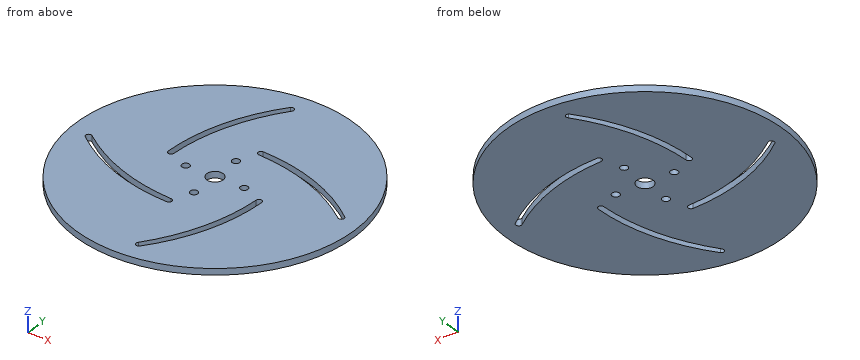
```python
from build123d import *

# Parameters (mm, degrees)
SKETCH1_R           = 69.85
SKETCH1_R_2         = 4.1
BOSS_EXTRUDE1_DEPTH = 3.175
SKETCH4_R           = 1.905
CUT_EXTRUDE1_DEPTH  = 4.175


with BuildPart() as part:
    # Sketch1 → Boss-Extrude1 (new body)
    with BuildSketch(Plane.XY):
        Circle(SKETCH1_R)
        Circle(SKETCH1_R_2, mode=Mode.SUBTRACT)
        with BuildLine():
            ThreePointArc((60.715904818, 5.788404818), (34.486591453, 20.94201271), (4.777601385, 26.856792578))
            ThreePointArc((4.777601385, 26.856792578), (3.305570957, 25.407474231), (4.762499202, 23.942975224))
            ThreePointArc((4.762499202, 23.942975224), (33.266012569, 17.981736248), (58.664095182, 3.736595182))
            ThreePointArc((58.664095182, 3.736595182), (60.715904818, 3.736595182), (60.715904818, 5.788404818))
        make_face(mode=Mode.SUBTRACT)
        with BuildLine():
            ThreePointArc((-23.942975224, 4.762499202), (-17.981736248, 33.266012569), (-3.736595182, 58.664095182))
            ThreePointArc((-3.736595182, 58.664095182), (-3.736595182, 60.715904818), (-5.788404818, 60.715904818))
            ThreePointArc((-5.788404818, 60.715904818), (-20.94201271, 34.486591453), (-26.856792578, 4.777601385))
            ThreePointArc((-26.856792578, 4.777601385), (-25.407474231, 3.305570957), (-23.942975224, 4.762499202))
        make_face(mode=Mode.SUBTRACT)
        with BuildLine():
            ThreePointArc((5.788404818, -60.715904818), (20.94201271, -34.486591453), (26.856792578, -4.777601385))
            ThreePointArc((26.856792578, -4.777601385), (25.407474231, -3.305570957), (23.942975224, -4.762499202))
            ThreePointArc((23.942975224, -4.762499202), (17.981736248, -33.266012569), (3.736595182, -58.664095182))
            ThreePointArc((3.736595182, -58.664095182), (3.736595182, -60.715904818), (5.788404818, -60.715904818))
        make_face(mode=Mode.SUBTRACT)
        with BuildLine():
            ThreePointArc((-60.715904818, -5.788404818), (-34.486591453, -20.94201271), (-4.777601385, -26.856792578))
            ThreePointArc((-4.777601385, -26.856792578), (-3.305570957, -25.407474231), (-4.762499202, -23.942975224))
            ThreePointArc((-4.762499202, -23.942975224), (-33.266012569, -17.981736248), (-58.664095182, -3.736595182))
            ThreePointArc((-58.664095182, -3.736595182), (-60.715904818, -3.736595182), (-60.715904818, -5.788404818))
        make_face(mode=Mode.SUBTRACT)
    extrude(amount=BOSS_EXTRUDE1_DEPTH)

    # Sketch4 → Cut-Extrude1 (cut, through all)
    with BuildSketch(Plane.XY.offset(3.175)):
        with Locations((14.605, 0)):
            Circle(SKETCH4_R)
        with Locations((0, -14.605)):
            Circle(SKETCH4_R)
        with Locations((-14.605, 0)):
            Circle(SKETCH4_R)
        with Locations((0, 14.605)):
            Circle(SKETCH4_R)
    extrude(amount=-CUT_EXTRUDE1_DEPTH, mode=Mode.SUBTRACT)


solid = part.part
```
Source: CAD feature listing. Evaluate the final solid. Frame: model axes, mm. Coordinates: 2 decimals unless noted, no trailing zeros. Loops run counter-clockwise (first coordinate to the right, second up) from the corner with the lowest first, then second, coordinate; pieces in that order, holes last. Notation, with made-up numbers: M 23,37 L 37,37 A9 ccw 37,46 Z; hole C -25.75,76.25 d2. An arc over 180 degrees is marked long. Use a Markdown table: item, result. Add a question column.
Q1. Material intervals for L1, parallel to Y at x = 0, z = 0.9; L2, parallel to Y at x = 6.5, z = 1.75; L3, parallel to X at y = 13, z = 2, sorted ascending.
Q2. Section query C-C, the plane z = 1.6. State how many separate pieces and enclosed holes the cut face has, and give its area (3 significant figures).
Q3. Section query D-D, the plane y = -29. Return loops of the section in (x, z) (3 decimals), and give its area (3 significant figures).
Q4. Section query A-A, the plane y = 0. Return loops of the section in (x, z) (3 decimals).
Q5. First-contact query: pin 1 (1 mm diameter, centred on x = 32, z = 0.5, fed in from +Y). Flat tip, straight axial feed; report the tip coordinate or a pass-through.
Result:
| question | item | result |
|---|---|---|
| 1 | L1 | y = -69.85 to -16.51, -12.7 to -4.1, 4.1 to 12.7, 16.51 to 69.85 |
| 1 | L2 | y = -69.55 to -59.84, -54.95 to 23.83, 26.78 to 69.55 |
| 1 | L3 | x = -68.63 to -26.22, -23.14 to -1.03, 1.03 to 44.36, 50.63 to 68.63 |
| 2 | separate pieces | 1 |
| 2 | enclosed holes | 9 |
| 2 | area | 14,500 mm2 |
| 3 | outline | M -63.545,0 L 19.467,0 L 19.467,3.175 L -63.545,3.175 Z; M 22.815,0 L 63.545,0 L 63.545,3.175 L 22.815,3.175 Z |
| 3 | area | 393 mm2 |
| 4 | outline | M -69.85,0 L -16.51,0 L -16.51,3.175 L -69.85,3.175 Z; M -12.7,0 L -4.1,0 L -4.1,3.175 L -12.7,3.175 Z; M 4.1,0 L 12.7,0 L 12.7,3.175 L 4.1,3.175 Z; M 16.51,0 L 69.85,0 L 69.85,3.175 L 16.51,3.175 Z |
| 5 | pin 1 | stops at y = 62.34 |
